```python
from build123d import *

# Parameters (mm, degrees)
EXTRUDE_1_DEPTH     = 8
CUT_EXTRUDE_1_DEPTH = 164.196200936
SKETCH_6_W          = 60.4
SKETCH_6_H          = 60.4
CUT_EXTRUDE_2_DEPTH = 164.196200936


with BuildPart() as part:
    # 草图2 → 凸台-拉伸1 (new body)
    with BuildSketch(Plane(origin=(0, 0, 0), x_dir=(1, 0, 0), z_dir=(0, 1, 0))):
        Polygon((-40, 28.686291501), (-40, 40), (-28.686291501, 40), (-103.944696834, 115.258405333), (-115.258405333, 103.944696834), align=None)
        Polygon((103.944696834, 115.258405333), (28.686291501, 40), (40, 40), (40, 28.686291501), (115.258405333, 103.944696834), align=None)
        Polygon((40, 10), (40, 40), (-40, 40), (-40, 10), (-30, 10), (-30, 30), (30, 30), (30, 10), align=None)
    extrude(amount=EXTRUDE_1_DEPTH)

    # 草图5 → 切除-拉伸1 (cut, through all)
    with BuildSketch(Plane(origin=(0, 8, 0), x_dir=(1, 0, 0), z_dir=(0, 1, 0))):
        Polygon((-105.783174466, 99.843477504), (-98.429263941, 92.489566979), (-92.489566979, 98.429263941), (-99.843477504, 105.783174466), align=None)
        Polygon((92.489566979, 98.429263941), (98.429263941, 92.489566979), (105.783174466, 99.843477504), (99.843477504, 105.783174466), align=None)
    extrude(amount=-CUT_EXTRUDE_1_DEPTH, mode=Mode.SUBTRACT)

    # 草图6 → 切除-拉伸2 (cut, through all)
    with BuildSketch(Plane(origin=(0, 8, 0), x_dir=(1, 0, 0), z_dir=(0, 1, 0))):
        Rectangle(SKETCH_6_W, SKETCH_6_H)
    extrude(amount=-CUT_EXTRUDE_2_DEPTH, mode=Mode.SUBTRACT)


solid = part.part
```
Input: part model. Units: mm. Frame: model coordinates. A direction names the side the tool comes from. Round coordinates to 2 decimals unless told otherwise and drop trailing zeros. Loops run counter-clockwise (first coordinate to the right, second up) from the corner with the lowest first, then second, coordinate; pieces in that order, holes last. Notation, with made-up numbers: (15.5, 1) - (32.5, 1) arc R9 cw to (32.5, 14) - close; hole circle Ø4 at (-4.5, -10.5). An arc over 180 degrees is marked (long way). One line per item, written item: value. Start each with the question number.
(1) Section D-D, the plane x = 12. Return loops of the section in (y, z), plus the area to 3 significant figures.
(2) Section C-C, the plane x = -95. Return loops of the section in (y, z).
(3) Ray query, line 1 (X direction, y = 4, z = -101.5); line 2 (X direction, y = 1.5, z = -93); line 3 (X direction, y = 1.25, z = -28.5). Return the intervals inside material, ascending. Write a range as [from, to].
(4) Section B-B, the plane y = 1.75. Return loops of the section in (x, z).
(5) Access query for faces 1 (the flat face through (0, 4, -40)), 2 (the flat face through (-96.115, 4.056, -102.055)), 3 (the flat face through (40, 4, -19)). Directions: +Z, -Z, +X, -X, +Y, -Y. A direction counts if a zero-diameter tool reaches every point of the face in a straight line with its end or side. Return the directions, or none.
(6) Contact query for flat-ended pins moving along their axis: P1, Ø1.5, axis at x = 28, y = 5, coming from the -Z side; P2, Ø4, axis at x = 4.5, y = 2, coming from the -Z side; P3, Ø1, axis at x = -79.5, y = 6, coming from the -Z side. Output: stop coordinate, or through.
(7) Section A-A, the plane z = -21. Return loops of the section in (x, y).
(8) Draft query along Z for faces 4 (the flat face through (-35, 4, -10)), 5 (the flat face through (-102.772, 4.056, -102.855)), 6 (the flat face through (102.055, 4.056, -96.115)), 7 (the flat face through (-1, 0, -36)). Return one class per face: +Z half, -Z half, draft (parallel to the pull), parting line (faces both ways), or undercut.
Results below:
1. outline: (0, -40) - (8, -40) - (8, -30.2) - (0, -30.2) - close
1. area: 78.4 mm^2
2. outline: (0, -106.31) - (8, -106.31) - (8, -100.94) - (0, -100.94) - close; (0, -95.92) - (8, -95.92) - (8, -83.69) - (0, -83.69) - close
3. line 1: [-112.81, -104.13], [-95.56, -90.19], [90.19, 95.56], [104.13, 112.81]
3. line 2: [-104.31, -98.94], [-97.92, -81.69], [81.69, 97.92], [98.94, 104.31]
3. line 3: [-40, -30.2], [30.2, 40]
4. outline: (-115.26, -103.94) - (-103.94, -115.26) - (-28.69, -40) - (28.69, -40) - (103.94, -115.26) - (115.26, -103.94) - (40, -28.69) - (40, -10) - (30.2, -10) - (30.2, -30.2) - (-30.2, -30.2) - (-30.2, -10) - (-40, -10) - (-40, -28.69) - close; hole (-105.78, -99.84) - (-99.84, -105.78) - (-92.49, -98.43) - (-98.43, -92.49) - close; hole (92.49, -98.43) - (99.84, -105.78) - (105.78, -99.84) - (98.43, -92.49) - close
5. face 1: -Z, +Y, -Y
5. face 2: +Y, -Y
5. face 3: +Z, +X, +Y, -Y
6. P1: z = -40.06
6. P2: z = -40
6. P3: z = -91.31
7. outline: (-40, 0) - (-30.2, 0) - (-30.2, 8) - (-40, 8) - close; (30.2, 0) - (40, 0) - (40, 8) - (30.2, 8) - close
8. face 4: +Z half
8. face 5: undercut
8. face 6: undercut
8. face 7: draft
